```python
from build123d import *

# Parameters (mm, degrees)
PAD007_DEPTH    = 5
POCKET016_DEPTH = 5
SKETCH028_R     = 3.15
POCKET_DEPTH    = 2
SKETCH041_R     = 1.3
POCKET024_DEPTH = 3


with BuildPart() as part:
    # Sketch025 → Pad007 (new body)
    with BuildSketch(Plane.XY):
        with BuildLine():
            Line((0, 28.5), (0, 57))
            Line((0, 57), (57, 57))
            Line((57, 57), (57, 28.5))
            ThreePointArc((0, 28.5), (28.5, 0), (57, 28.5))
        make_face()
    extrude(amount=PAD007_DEPTH)

    # Sketch026 (on Face6 of Pad007) → Pocket016 (cut)
    with BuildSketch(Plane.XY.offset(5)):
        Polygon((22.5, 15), (34.5, 15), (34.5, 24), (45, 24), (45, 44), (80.717206, 57), (45, 57), (12, 57), (-23.717206, 57), (12, 44), (12, 24), (22.5, 24), align=None)
    extrude(amount=-POCKET016_DEPTH, mode=Mode.SUBTRACT)

    # Sketch028 (on Face4 of Pocket016) → Pocket (cut)
    with BuildSketch(Plane.XY.offset(5)):
        with Locations((19.5, 7.5)):
            Circle(SKETCH028_R)
        with Locations((37.5, 7.5)):
            Circle(SKETCH028_R)
    extrude(amount=-POCKET_DEPTH, mode=Mode.SUBTRACT)

    # Sketch041 (on Face18 of Pocket) → Pocket024 (cut)
    with BuildSketch(Plane.XY.offset(3)):
        with Locations((19.5, 7.5)):
            Circle(SKETCH041_R)
        with Locations((37.5, 7.5)):
            Circle(SKETCH041_R)
    extrude(amount=-POCKET024_DEPTH, mode=Mode.SUBTRACT)


solid = part.part
```
Can you work these out from the model? Positions are in its coordinate system, mm. A direction names the side the tool comes from. Coordinates: 2 decimals unless noted, no trailing zeros. Loops run counter-clockwise (first coordinate to the right, second up) from the corner with the lowest first, then second, coordinate; pieces in that order, holes last. Notation, with made-up numbers: (68.25, 33.25) -> (118.25, 33.25) arc R22 cw to (118.25, 40.25) -> close; hole circle Ø10 at (68.5, 10). An arc over 180 degrees is marked (long way). Put each result on its own line as item: value. Start each with the question number.
Q1. I want a section at B-B (z = 4.4). Write out the boundary of the cut face in (x, y).
Q2. I want a section at C-C (y = 7.5). Write out the boundary of the cut face in (x, z).
Q3. If I drill on line 1 (X direction, y = 32.5, z = 3.65); line 2 (Y direction, x = 40, z = 3.6); line 3 (Y direction, x = 38, z = 0.85), over which ranges is the centre line in solid material (lowest first)? Write a range as [from, to].
Q4. I want a section at D-D (x = 37.5). Write out the boundary of the cut face in (y, z), plus the area to 3 significant figures.
Q5. Thinking about a two-plate mould opening in X: for faces 1 (the face through (35, 19, 0)), 2 (the face through (57, 39, 2)), 3 (the face through (0, 38, 2)), 4 (the face through (18.2, 7.56, 1.52)), which applies, pulls with the +X half, pulls with the -X half, needs draft (parallel to the pull), parting line crosses it, or undercut?
Q6. I'm going to push flat-ended pins straight in: P1, Ø1.5, axis at x = 37.5, z = 3.5, coming from the +Y side; P2, Ø2.5, axis at y = 17.5, z = 3.5, coming from the -X side. Where does each tip first touch, or does it pass through?
Q7. I want a section at A-A (y = 34). Write out the boundary of the cut face in (x, z).
Q8. For faces 5 (the face through (50.916, 46.153, 2.535)), 6 (the face through (27.873, 0.007, 2.465)), 7 (the face through (19.09, 10.623, 4.014)), which set-ups out of +Z, -Z, +X, -X, +Y, -Y let a thin tool reach every point of the face, with its end or its side?
Taken from the geometry:
1. outline: (0, 28.5) arc R28.5 ccw to (57, 28.5) -> (57, 48.37) -> (45, 44) -> (45, 24) -> (34.5, 24) -> (34.5, 15) -> (22.5, 15) -> (22.5, 24) -> (12, 24) -> (12, 44) -> (0, 48.37) -> close; hole circle Ø6.3 at (19.5, 7.5); hole circle Ø6.3 at (37.5, 7.5)
2. outline: (9.23, 0) -> (18.2, 0) -> (18.2, 3) -> (16.35, 3) -> (16.35, 5) -> (9.23, 5) -> close; (20.8, 0) -> (36.2, 0) -> (36.2, 3) -> (34.35, 3) -> (34.35, 5) -> (22.65, 5) -> (22.65, 3) -> (20.8, 3) -> close; (38.8, 0) -> (47.77, 0) -> (47.77, 5) -> (40.65, 5) -> (40.65, 3) -> (38.8, 3) -> close
3. line 1: x = [0, 12], [45, 57]
3. line 2: y = [2.42, 5.58], [9.42, 24]
3. line 3: y = [1.63, 6.3], [8.7, 24]
4. outline: (1.46, 0) -> (6.2, 0) -> (6.2, 3) -> (4.35, 3) -> (4.35, 5) -> (1.46, 5) -> close; (8.8, 0) -> (24, 0) -> (24, 5) -> (10.65, 5) -> (10.65, 3) -> (8.8, 3) -> close
4. area: 92.3 mm2
5. face 1: needs draft
5. face 2: pulls with the +X half
5. face 3: pulls with the -X half
5. face 4: undercut
6. P1: stops at y = 24
6. P2: stops at x = 1.72
7. outline: (0, 0) -> (12, 0) -> (12, 5) -> (0, 5) -> close; (45, 0) -> (57, 0) -> (57, 5) -> (45, 5) -> close
8. face 5: +Z, -Z, +Y
8. face 6: +Z, -Z, -Y
8. face 7: +Z
